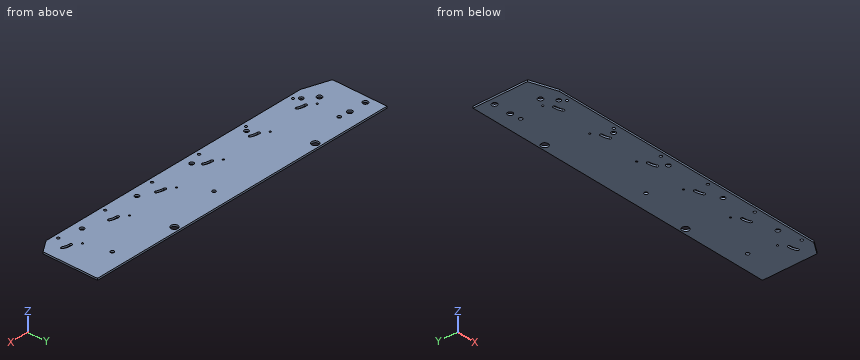
from build123d import *

# Parameters (mm, degrees)
EXTRUDE_1_DEPTH        = 2
SKETCH_2_R             = 1.5
CUT_EXTRUDE_1_DEPTH    = 2
PATTERN_LINEAR_1_COUNT = 6
PATTERN_LINEAR_1_PITCH = 60
SKETCH_3_R             = 2.5
CUT_EXTRUDE_2_DEPTH    = 2
PATTERN_LINEAR_2_COUNT = 5
PATTERN_LINEAR_2_PITCH = 70
SKETCH_4_R             = 2
CUT_EXTRUDE_3_DEPTH    = 2
CUT_EXTRUDE_5_REACH    = 4
SKETCH_6_R             = 3
CUT_EXTRUDE_6_DEPTH    = 2
PATTERN_LINEAR_3_COUNT = 6
PATTERN_LINEAR_3_PITCH = 60
SKETCH_8_R             = 1
CUT_EXTRUDE_7_DEPTH    = 2
PATTERN_LINEAR_4_COUNT = 6
PATTERN_LINEAR_4_PITCH = 60
SKETCH_9_W             = 370
SKETCH_9_H             = 13
EXTRUDE_2_DEPTH        = 2
SKETCH_10_R            = 4
CUT_EXTRUDE_8_DEPTH    = 2


with BuildPart() as part:
    # 草图1 → 凸台-拉伸1 (new body)
    with BuildSketch(Plane.XY):
        Polygon((-162.5, 0), (162.5, 0), (177.5, 10), (177.5, 60), (-192.5, 60), (-192.5, 10), align=None)
    extrude(amount=EXTRUDE_1_DEPTH)

    # 草图2 → 切除-拉伸1 (cut)
    with BuildSketch(Plane.XY.offset(2)):
        with Locations((-147.5, 5)):
            Circle(SKETCH_2_R)
    cut_extrude_1 = extrude(amount=-CUT_EXTRUDE_1_DEPTH, mode=Mode.SUBTRACT)

    # 阵列(线性)1: 切除-拉伸1 ×6
    with Locations(*[(i * PATTERN_LINEAR_1_PITCH, 0, 0) for i in range(1, PATTERN_LINEAR_1_COUNT)]):
        add(cut_extrude_1, mode=Mode.SUBTRACT)

    # 草图3 → 切除-拉伸2 (cut)
    with BuildSketch(Plane.XY.offset(2)):
        with Locations((-152.5, 10)):
            Circle(SKETCH_3_R)
    cut_extrude_2 = extrude(amount=-CUT_EXTRUDE_2_DEPTH, mode=Mode.SUBTRACT)

    # 阵列(线性)2: 切除-拉伸2 ×5
    with Locations(*[(i * PATTERN_LINEAR_2_PITCH, 0, 0) for i in range(1, PATTERN_LINEAR_2_COUNT)]):
        add(cut_extrude_2, mode=Mode.SUBTRACT)

    # 草图4 → 切除-拉伸3 (cut)
    with BuildSketch(Plane.XY.offset(2)):
        with Locations((-152.5, 54)):
            Circle(SKETCH_4_R)
        with Locations((7.5, 54)):
            Circle(SKETCH_4_R)
        with Locations((137.5, 54)):
            Circle(SKETCH_4_R)
    extrude(amount=-CUT_EXTRUDE_3_DEPTH, mode=Mode.SUBTRACT)

    # 草图6 → 切除-拉伸5 (cut, up to next)
    with BuildSketch(Plane.XY.offset(2), mode=Mode.PRIVATE) as cut_extrude_5_sk1:
        with Locations((-184.57, 55.21)):
            Circle(SKETCH_6_R)
    cut_extrude_5_tool1 = extrude(cut_extrude_5_sk1.sketch, amount=-CUT_EXTRUDE_5_REACH, mode=Mode.PRIVATE) & part.part
    add(cut_extrude_5_tool1.solids().sort_by_distance((-184.57, 55.21, 2))[0], mode=Mode.SUBTRACT)
    # 草图6 → 切除-拉伸5 (cut, up to next)
    with BuildSketch(Plane.XY.offset(2), mode=Mode.PRIVATE) as cut_extrude_5_sk2:
        with Locations((-164.57, 55.21)):
            Circle(SKETCH_6_R)
    cut_extrude_5_tool2 = extrude(cut_extrude_5_sk2.sketch, amount=-CUT_EXTRUDE_5_REACH, mode=Mode.PRIVATE) & part.part
    add(cut_extrude_5_tool2.solids().sort_by_distance((-164.57, 55.21, 2))[0], mode=Mode.SUBTRACT)
    # 草图6 → 切除-拉伸5 (cut, up to next)
    with BuildSketch(Plane.XY.offset(2), mode=Mode.PRIVATE) as cut_extrude_5_sk3:
        with Locations((-164.57, 20.21)):
            Circle(SKETCH_6_R)
    cut_extrude_5_tool3 = extrude(cut_extrude_5_sk3.sketch, amount=-CUT_EXTRUDE_5_REACH, mode=Mode.PRIVATE) & part.part
    add(cut_extrude_5_tool3.solids().sort_by_distance((-164.57, 20.21, 2))[0], mode=Mode.SUBTRACT)

    # 草图7 → 切除-拉伸6 (cut)
    with BuildSketch(Plane.XY.offset(2)):
        with BuildLine():
            ThreePointArc((-147.22, 21.5), (-148.72, 20), (-147.22, 18.5))
            ThreePointArc((-147.22, 18.5), (-143.000780895, 18.012446152), (-139.003950762, 16.575481472))
            ThreePointArc((-139.003950762, 16.575481472), (-136.993826903, 17.253273526), (-137.671618958, 19.263397386))
            ThreePointArc((-137.671618958, 19.263397386), (-142.316583462, 20.933383309), (-147.22, 21.5))
        make_face()
    cut_extrude_6 = extrude(amount=-CUT_EXTRUDE_6_DEPTH, mode=Mode.SUBTRACT)

    # 阵列(线性)3: 切除-拉伸6 ×6
    with Locations(*[(i * PATTERN_LINEAR_3_PITCH, 0, 0) for i in range(1, PATTERN_LINEAR_3_COUNT)]):
        add(cut_extrude_6, mode=Mode.SUBTRACT)

    # 草图8 → 切除-拉伸7 (cut)
    with BuildSketch(Plane.XY.offset(2)):
        with Locations((-155.22, 26)):
            Circle(SKETCH_8_R)
    cut_extrude_7 = extrude(amount=-CUT_EXTRUDE_7_DEPTH, mode=Mode.SUBTRACT)

    # 阵列(线性)4: 切除-拉伸7 ×6
    with Locations(*[(i * PATTERN_LINEAR_4_PITCH, 0, 0) for i in range(1, PATTERN_LINEAR_4_COUNT)]):
        add(cut_extrude_7, mode=Mode.SUBTRACT)

    # 草图9 → 凸台-拉伸2 (add)
    with BuildSketch(Plane.XY):
        with Locations((-7.5, 66.5)):
            Rectangle(SKETCH_9_W, SKETCH_9_H)
    extrude(amount=EXTRUDE_2_DEPTH)

    # 草图10 → 切除-拉伸8 (cut)
    with BuildSketch(Plane.XY.offset(2)):
        with Locations((-107.5, 67)):
            Circle(SKETCH_10_R)
        with Locations((72.5, 67)):
            Circle(SKETCH_10_R)
    extrude(amount=-CUT_EXTRUDE_8_DEPTH, mode=Mode.SUBTRACT)


solid = part.part
Check sheet for the modelled part. Datum: model origin and axes. Units: mm. Round coordinates to 2 decimals unless told otherwise and drop trailing zeros. Order: outer loops, then holes, each group sorted by start corner. A loop starts at its lowest first (then second) coordinate and runs counter-clockwise, first axis right, second up. Notation, with made-up numbers: M 48,64.5 L 76,64.5 A9 ccw 76,68.5 Z; hole C -9,-18.5 d10. An arc over 180 degrees is marked long. One line per item, written item: value. Start each with the question number.
1. Section check B-B on z = 0.85. Give the number of separate pieces and of enclosed holes in the cut face, and give its area (3 significant figures).
2. Scan lines: line 1 along X through (y, z) = (57, 1.1); line 2 along Y through (x, z) = (-164.57, 1.5); line 3 along Y through (x, z) = (-107.5, 0.8). Record each from-to range of solid material in increasing order.
3. Gauge pin test, flat end, axial feed: P1, Ø1.8, axis at x = -35.22, y = 26, coming from the -Z side. Record the tip position at first contact, or that the pin passes through.
4. Section check A-A on x = 72.5. Enter the section's corners in (y, z).
Results found:
1. separate pieces: 1
1. enclosed holes: 31
1. area: 26,200 mm^2
2. line 1: -192.5 to -186.98, -182.16 to -166.98, -162.16 to 177.5
2. line 2: 0.69 to 17.21, 23.21 to 52.21, 58.21 to 73
2. line 3: 0 to 63, 71 to 73
3. P1: through
4. outline: M 0,0 L 63,0 L 63,2 L 0,2 Z; M 71,0 L 73,0 L 73,2 L 71,2 Z
